The listing builds one solid part. Answer for the finished solid, in the listing's coordinates (mm). Face numbers are marked on the shaded views. A direction names the side the tool comes from. Give positions to 0.01 mm unless a question says otherwise; leave off trailing zeros. Loops run counter-clockwise (first coordinate to the right, second up) from the corner with the lowest first, then second, coordinate; pieces in that order, holes last. Notation, with made-up numbers: (20.25, 54) - (37.25, 54) arc R16 cw to (37.25, 78) - close; hole circle Ø6 at (67, 27.25). An arc over 180 degrees is marked (long way). One line per item, written item: value. Start each with the question number.
from build123d import *

# Parameters (mm, degrees)
EXTRUDE_1_DEPTH     = 42
FILLET_1_R          = 2
FILLET_2_R          = 1
FILLET_3_R          = 1
CUT_EXTRUDE_1_REACH = 89.88
SKETCH_2_R          = 4.25
CUT_EXTRUDE_2_REACH = 94.906
SKETCH_3_R          = 4.25
SKETCH_4_W          = 42
SKETCH_4_H          = 1
CUT_EXTRUDE_3_DEPTH = 0.2
SKETCH_5_W          = 1
SKETCH_5_H          = 42
CUT_EXTRUDE_4_DEPTH = 0.2


with BuildPart() as part:
    # 草图1 → 凸台-拉伸1 (new body)
    with BuildSketch(Plane.XY):
        Polygon((0, 0), (60, 0), (60, 8), (40, 8), (28.083261121, 36.769552622), (42.225396744, 50.911688245), (36.568542495, 56.568542495), (-20, 0), align=None)
        with BuildLine():
            Line((24.130306277, 38.473452028), (2.067060132, 16.410205883))
            ThreePointArc((2.067060132, 16.410205883), (3.161356319, 14.825706508), (4.142085372, 13.168512212))
            ThreePointArc((4.142085372, 13.168512212), (5.535917687, 13.696629788), (7.01188026, 13.488756805))
            ThreePointArc((7.01188026, 13.488756805), (7.256435362, 12.901225698), (6.668904255, 12.656670595))
            ThreePointArc((6.668904255, 12.656670595), (3.928479892, 9.911500898), (7.80738065, 9.90814544))
            ThreePointArc((7.80738065, 9.90814544), (8.395754452, 10.150666099), (8.638275111, 9.562292298))
            ThreePointArc((8.638275111, 9.562292298), (7.741600362, 8.371640758), (6.382576562, 7.759487995))
            ThreePointArc((6.382576562, 7.759487995), (6.860909722, 5.894194507), (7.207535721, 4))
            Line((7.207535721, 4), (38.409677649, 4))
            Line((38.409677649, 4), (24.130306277, 38.473452028))
        make_face(mode=Mode.SUBTRACT)
        with BuildLine():
            Line((-10.343145751, 4), (4.677925359, 4))
            ThreePointArc((4.677925359, 4), (3.096988313, 9.567085809), (0.278355491, 14.621501242))
            Line((0.278355491, 14.621501242), (-10.343145751, 4))
        make_face(mode=Mode.SUBTRACT)
    extrude(amount=EXTRUDE_1_DEPTH)

    # 圆角1
    fillet_1_edges = [part.edges().sort_by_distance(p)[0] for p in [
        (-20, 0, 21),
    ]]
    fillet(fillet_1_edges, radius=FILLET_1_R)

    # 圆角2
    fillet_2_edges = [part.edges().sort_by_distance(p)[0] for p in [
        (-10.343145751, 4, 21),
    ]]
    fillet(fillet_2_edges, radius=FILLET_2_R)

    # 圆角3
    fillet_3_edges = [part.edges().sort_by_distance(p)[0] for p in [
        (38.409677649, 4, 21),
        (24.130306277, 38.473452028, 21),
    ]]
    fillet(fillet_3_edges, radius=FILLET_3_R)

    # 草图2 → 切除-拉伸1 (cut, up to next)
    with BuildSketch(Plane(origin=(0, 8, 0), x_dir=(1, 0, 0), z_dir=(0, 1, 0)), mode=Mode.PRIVATE) as cut_extrude_1_sk1:
        with Locations(Location((50, -21, 0), (0, 0, 270))):
            Circle(SKETCH_2_R)
    cut_extrude_1_tool1 = extrude(cut_extrude_1_sk1.sketch, amount=-CUT_EXTRUDE_1_REACH, mode=Mode.PRIVATE) & part.part
    add(cut_extrude_1_tool1.solids().sort_by_distance((50, 8, 21))[0], mode=Mode.SUBTRACT)

    # 草图3 → 切除-拉伸2 (cut, up to next)
    with BuildSketch(Plane(origin=(-4.343145751, 4.343145751, 0), x_dir=(0, 0, -1), z_dir=(0.7071067811865441, -0.7071067811865509, 0)), mode=Mode.PRIVATE) as cut_extrude_2_sk1:
        with Locations(Location((-21, 55.857864376, 0), (0, 0, 90))):
            Circle(SKETCH_3_R)
    cut_extrude_2_tool1 = extrude(cut_extrude_2_sk1.sketch, amount=-CUT_EXTRUDE_2_REACH, mode=Mode.PRIVATE) & part.part
    add(cut_extrude_2_tool1.solids().sort_by_distance((35.154329, 43.84062, 21))[0], mode=Mode.SUBTRACT)

    # 草图4 → 切除-拉伸3 (cut)
    with BuildSketch(Plane(origin=(-4.343145751, 4.343145751, 0), x_dir=(0, 0, -1), z_dir=(0.7071067811865441, -0.7071067811865509, 0))):
        with Locations((-21, 55.857864376)):
            Rectangle(SKETCH_4_W, SKETCH_4_H)
    extrude(amount=-CUT_EXTRUDE_3_DEPTH, mode=Mode.SUBTRACT)

    # 草图5 → 切除-拉伸4 (cut)
    with BuildSketch(Plane(origin=(0, 8, 0), x_dir=(1, 0, 0), z_dir=(0, 1, 0))):
        with Locations((50, -21)):
            Rectangle(SKETCH_5_W, SKETCH_5_H)
    extrude(amount=-CUT_EXTRUDE_4_DEPTH, mode=Mode.SUBTRACT)


solid = part.part
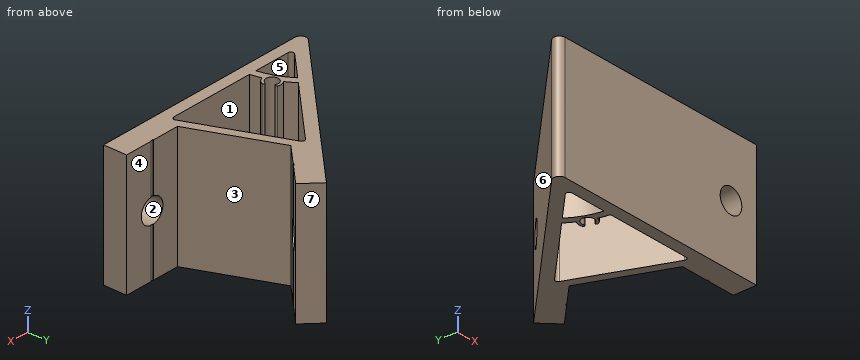
1. Flat-ended cylindrical pins translate along their axes: pin 1 (0.8 mm diameter, centred on x = 50, z = 35.5, fed in from +Y); pin 2 (5 mm diameter, centred on y = 18.5, z = 37.5, fed in from +X); pin 3 (2 mm diameter, centred on x = 12.5, z = 21.5, fed in from +Y). Find the tip coordinate at first contact, or state that the pin passes through.
2. A cutting plane is placed at A-A (z = 22). Give the number of separate pieces and of enclosed holes in the cut face, plus the area to 3 significant figures.
3. A cutting plane is placed at D-D (y = 39.5). Determine the outline of the cut face in (x, z).
4. For the marked faces 1, 2 and 3, determine the directions among +Z, -Z, +X, -X, +Y, -Y from which every point of the face is accessible in a straight line to the end or side of a thin tool.
5. Determine the mould class of the marked faces 4, 5, 6 and 7 for opening direction X: released by +X, released by -X, zero draft, split by the parting line, or undercut.
6. Find the intervals of material crossed by L1, parallel to X at y = 2, z = 21; L2, parallel to Z at x = 50, y = 5; L3, parallel to Y at x = 34.5, z = 24, in increasing order. Write a range as [from, to].
7. A cutting plane is placed at B-B (y = 23). Determine the outline of the cut face in (x, z), plus the area to 3 significant figures.
Results below:
1. pin 1: stops at y = 7.8
1. pin 2: stops at x = 36.69
1. pin 3: stops at y = 33.5
2. separate pieces: 3
2. enclosed holes: 2
2. area: 768 mm^2
3. outline: (19.5, 0) - (30.81, 0) - (30.81, 42) - (19.5, 42) - close
4. face 1: +Z, -Z
4. face 2: +Y, -Y
4. face 3: +Z, -Z, +X
5. face 4: zero draft
5. face 5: undercut
5. face 6: released by -X
5. face 7: released by +X
6. L1: x = [-17.17, 45.75], [54.25, 60]
6. L2: z = [0, 16.75], [25.25, 42]
6. L3: y = [0, 4], [13.44, 21.28], [48.75, 54.5]
7. outline: (3, 0) - (8.66, 0) - (8.66, 42) - (3, 42) - close; (30.54, 0) - (33.79, 0) - (33.79, 42) - (30.54, 42) - close
7. area: 374 mm^2
